from build123d import *

# Parameters (mm, degrees)
STOCK_FRAME_1_START       = 97.5
STOCK_FRAME_1_DEPTH       = 10
STOCK_FRAME_1_START_2     = 100.5
STOCK_FRAME_1_2_OUTLINE_R = 0.7
STOCK_FRAME_1_2_OUTLINE_W = 23
STOCK_FRAME_1_2_OUTLINE_H = 12.65
STOCK_FRAME_1_2_DEPTH     = 7
CUT_EXTRUDE1_DEPTH        = 128.596397383
CUT_EXTRUDE1_DEPTH_BACK   = 128.596397383
SKETCH1_W                 = 49.919710218
SKETCH1_H                 = 2
CUT_EXTRUDE2_DEPTH        = 10
FILLET1_R                 = 0.5


# Read off the part's stored shape, not the designer's step: Stock-frame-1
with BuildPart() as part:
    # Stock-frame-1 outline → Stock-frame-1 (new body)
    with BuildSketch(Plane.YZ.offset(STOCK_FRAME_1_START)):
        with BuildLine():
            Line((-4.096596213, 2.525), (-38.259818101, 2.525))
            Line((-38.259818101, 2.525), (-38.259818101, 16.525))
            Line((-38.259818101, 16.525), (-4.096596213, 16.525))
            ThreePointArc((-4.096596213, 16.525), (-6.783664239, 18.601647078), (-10, 19.69159292))
            Line((-10, 19.69159292), (-124.3, 27.025))
            Line((-124.3, 27.025), (-124.3, -7.975))
            Line((-124.3, -7.975), (-10, -0.64159292))
            ThreePointArc((-10, -0.64159292), (-6.783664239, 0.448352922), (-4.096596213, 2.525))
        make_face()
        with BuildLine():
            ThreePointArc((-109.3, 16.915787193), (-108.668190305, 18.374572746), (-107.17194471, 18.911683443))
            Line((-107.17194471, 18.911683443), (-105.052772964, 18.775718884))
            ThreePointArc((-105.052772964, 18.775718884), (-104.356669901, 18.602118716), (-103.766614692, 18.194036196))
            Line((-103.766614692, 18.194036196), (-90.131771322, 4.559192826))
            ThreePointArc((-90.131771322, 4.559192826), (-89.674659008, 2.439189307), (-91.417929594, 1.149083013))
            Line((-91.417929594, 1.149083013), (-107.17194471, 0.138316557))
            ThreePointArc((-107.17194471, 0.138316557), (-108.668190305, 0.675427254), (-109.3, 2.134212807))
            Line((-109.3, 2.134212807), (-109.3, 16.915787193))
        make_face(mode=Mode.SUBTRACT)
        with BuildLine():
            ThreePointArc((-49.680780162, 15.223091028), (-48.224999236, 14.448449394), (-47.845976598, 12.84354765))
            ThreePointArc((-47.845976598, 12.84354765), (-48.167247509, 9.525), (-47.845976598, 6.20645235))
            ThreePointArc((-47.845976598, 6.20645235), (-48.224999236, 4.601550606), (-49.680780162, 3.826908972))
            Line((-49.680780162, 3.826908972), (-76.799489195, 2.0869918))
            ThreePointArc((-76.799489195, 2.0869918), (-77.633334442, 2.211562173), (-78.341758047, 2.668674488))
            Line((-78.341758047, 2.668674488), (-89.972181694, 14.299098134))
            ThreePointArc((-89.972181694, 14.299098134), (-90.380264213, 16.53747005), (-88.429912841, 17.709207947))
            Line((-88.429912841, 17.709207947), (-49.680780162, 15.223091028))
        make_face(mode=Mode.SUBTRACT)
    extrude(amount=STOCK_FRAME_1_DEPTH)

    # Stock-frame-1 2 outline → Stock-frame-1 2 (add)
    with BuildSketch(Plane.YZ.offset(STOCK_FRAME_1_START_2)):
        with BuildLine():
            Line((-38.259818101, 16.525), (-38.259818101, 2.525))
            Line((-38.259818101, 2.525), (-4.096596213, 2.525))
            ThreePointArc((-4.096596213, 2.525), (-1.352388693, 9.525), (-4.096596213, 16.525))
            Line((-4.096596213, 16.525), (-38.259818101, 16.525))
        make_face()
        with Locations((-35.059818101, 9.525)):
            Circle(STOCK_FRAME_1_2_OUTLINE_R, mode=Mode.SUBTRACT)
        with Locations((-21.259818101, 9.525)):
            Rectangle(STOCK_FRAME_1_2_OUTLINE_W, STOCK_FRAME_1_2_OUTLINE_H, mode=Mode.SUBTRACT)
        with Locations((-7.459818101, 9.525)):
            Circle(STOCK_FRAME_1_2_OUTLINE_R, mode=Mode.SUBTRACT)
    extrude(amount=STOCK_FRAME_1_2_DEPTH)

    # Sketch1 → Cut-Extrude1 (cut, two sides: drawn at the far end of the back side and taken through both)
    with BuildSketch(Plane(origin=(107.5, 0, 0), x_dir=(0, 0, -1), z_dir=(1, 0, 0)).offset(-CUT_EXTRUDE1_DEPTH_BACK)):
        with Locations((-2.065144891, -123.3)):
            Rectangle(SKETCH1_W, SKETCH1_H)
    extrude(amount=CUT_EXTRUDE1_DEPTH + CUT_EXTRUDE1_DEPTH_BACK, mode=Mode.SUBTRACT)

    # Sketch2 → Cut-Extrude2 (cut)
    with BuildSketch(Plane.XZ.offset(122.3)):
        Polygon((97.5, 12.525), (103.5, 14.525), (103.5, 4.525), (97.5, 6.525), align=None)
    extrude(amount=-CUT_EXTRUDE2_DEPTH, mode=Mode.SUBTRACT)

    # Fillet1
    fillet1_edges = [part.edges().sort_by_distance(p)[0] for p in [
        (97.5, -117.3, 6.525),
        (97.5, -117.3, 12.525),
    ]]
    fillet(fillet1_edges, radius=FILLET1_R)


solid = part.part
Verification items for the finished model (mm, model axes). A direction names the side the tool comes from. Coordinates: 2 decimals unless noted, no trailing zeros. Order: outer loops, then holes, each group sorted by start corner. A loop starts at its lowest first (then second) coordinate and runs counter-clockwise, first axis right, second up. Notation, with made-up numbers: M 73,62 L 111,62 A4 cw 111,68 Z; hole C 30.5,85.5 d7. An arc over 180 degrees is marked long. One line per item, written item: value. Start each with the question number.
Item 1: Sectioned sample at A-A on y = -94.5. Record the cut outline in (x, z).
Item 2: Mould release check, pull along X, two halves, no side actions. Record for faces 4 (the flat face through (100.79, -117.37, 13.62)), 5 (the flat face through (102.43, -97.04, 11.47)), 6 (the flat face through (103.5, -117, 10)): pulls with the +X half, pulls with the -X half, needs draft (parallel to the pull), parting line crosses it, or undercut.
Item 3: Access from +Z, -Z, +X, -X, +Y, -Y to the whole of each face (thin tool, end or side, straight path). Record for faces 1 (the cylindrical face through (102.43, -89.664, 2.469)), 2 (the flat face through (99, -21, 16.525)), 3 (the flat face through (101, -112.3, 10)).
Item 4: Sectioned sample at B-B on x = 102. Give the number of separate pieces and of enclosed holes in the cut face, then the cut area to 3 significant figures.
Item 5: Depth check by flat-ended pin: P1, Ø3.5, axis at x = 103, y = -26, coming from the +Z side; P2, Ø1.5, axis at x = 98.5, z = 14.5, coming from the +Y side; P3, Ø4, axis at x = 99.5, y = -85.5, coming from the -Z side. Enter the tip coordinate at first touch or a pass-through.
Item 6: Thickness scan on probe 1 along Y at (x, z) = (104.25, 8); probe 2 along Y at (x, z) = (100.25, 5.5); probe 3 along Y at (x, z) = (103.25, 7.5). Record the ranges inside material, lowest first.
Item 7: Sectioned sample at D-D on y = -25.5. Record the cut outline in (x, z) (3 decimals), then the cut area to 3 significant figures.
Item 8: Sectioned sample at C-C on y = -114.5. Record the cut outline in (x, z) (3 decimals), then the cut area to 3 significant figures.
Calculated:
1. outline: M 97.5,-6.06 L 107.5,-6.06 L 107.5,0.95 L 97.5,0.95 Z; M 97.5,8.93 L 107.5,8.93 L 107.5,25.11 L 97.5,25.11 Z
2. face 4: undercut
2. face 5: needs draft
2. face 6: undercut
3. face 1: +X, -X
3. face 2: -X, +Y
3. face 3: -Y
4. separate pieces: 1
4. enclosed holes: 5
4. area: 2,090 mm^2
5. P1: z = 20.83
5. P2: y = -38.26
5. P3: z = -5.61
6. probe 1: -122.3 to -109.3, -93.57 to -83.67, -48.1 to -32.76, -9.76 to -1.47
6. probe 2: -122.3 to -109.3, -91.07 to -81.17, -47.84 to -38.26
6. probe 3: -112.3 to -109.3, -93.07 to -83.17, -48.05 to -32.76, -9.76 to -1.55
7. outline: M 97.5,-1.636 L 107.5,-1.636 L 107.5,3.2 L 100.5,3.2 L 100.5,2.525 L 97.5,2.525 Z; M 97.5,16.525 L 100.5,16.525 L 100.5,15.85 L 107.5,15.85 L 107.5,20.686 L 97.5,20.686 Z
7. area: 92.7 mm^2
8. outline: M 97.5,-7.346 L 107.5,-7.346 L 107.5,26.396 L 97.5,26.396 L 97.5,13.219 A0.5 ccw 98.158,12.744 L 103.5,14.525 L 103.5,4.525 L 98.158,6.306 A0.5 ccw 97.5,5.831 Z
8. area: 289 mm^2
